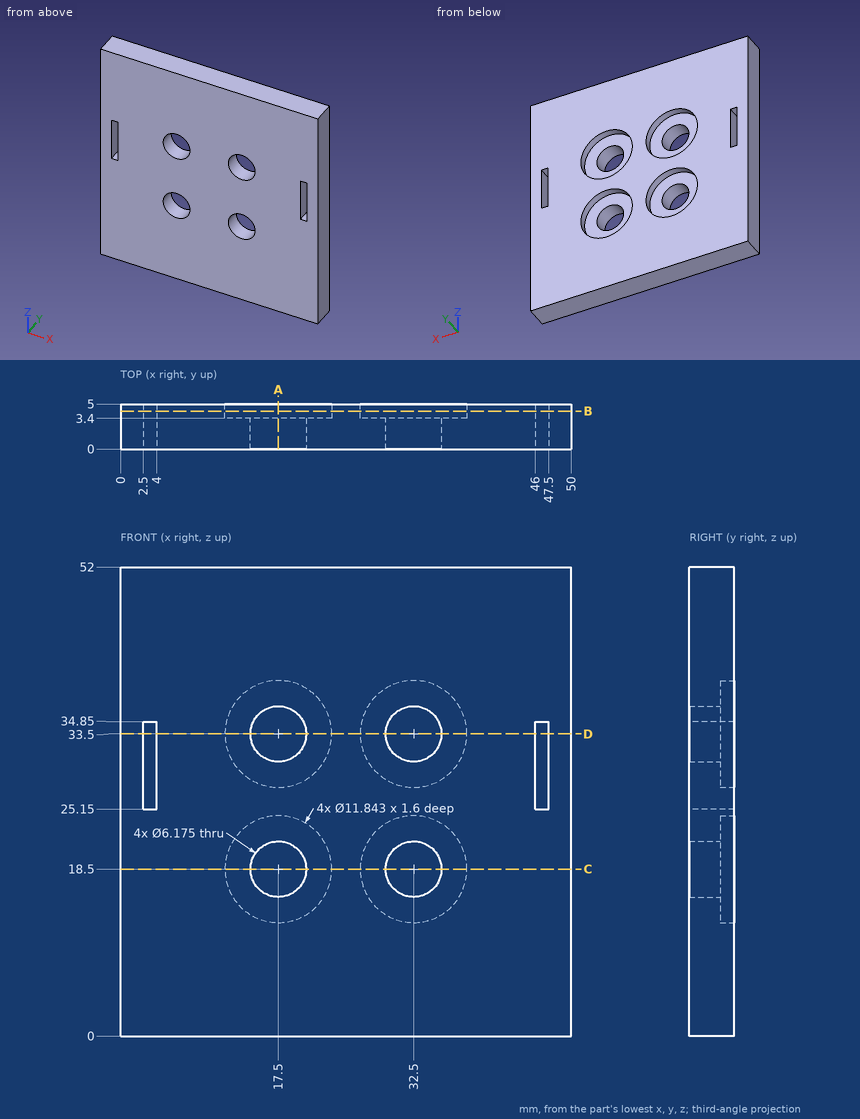
Design review of the part shown in the three views and the two pictorial views. Dimensions are in mm from the part's minimum x, y and z. Round coordinates to 2 decimals unless told otherwise and drop trailing zeros. Order: outer loops, then holes, each group sorted by start corner. A loop starts at its lowest first (then second) coordinate and runs counter-clockwise, first axis right, second up. Notation, with made-up numbers: M 12,-0.5 L 38,-0.5 A11 cw 38,16.5 Z; hole C -36,-32 d8. An arc over 180 degrees is marked long. Put each result on its own line as item: value.
Q1. Consider section A-A (x = 17.5). State the section outline as (y, z) points, and give its area (3 significant figures).
Reported:
outline: M 0,0 L 5,0 L 5,12.58 L 3.4,12.58 L 3.4,15.41 L 0,15.41 Z; M 0,21.59 L 3.4,21.59 L 3.4,24.42 L 5,24.42 L 5,27.58 L 3.4,27.58 L 3.4,30.41 L 0,30.41 Z; M 0,36.59 L 3.4,36.59 L 3.4,39.42 L 5,39.42 L 5,52 L 0,52 Z
area: 180 mm²
Q2. Consider section D-D (z = 33.5). State the section outline as (x, y) points, and give its area (3 significant figures).
Reported:
outline: M 0,0 L 2.5,0 L 2.5,5 L 0,5 Z; M 4,0 L 14.41,0 L 14.41,3.4 L 11.58,3.4 L 11.58,5 L 4,5 Z; M 20.59,0 L 29.41,0 L 29.41,3.4 L 26.58,3.4 L 26.58,5 L 23.42,5 L 23.42,3.4 L 20.59,3.4 Z; M 35.59,0 L 46,0 L 46,5 L 38.42,5 L 38.42,3.4 L 35.59,3.4 Z; M 47.5,0 L 50,0 L 50,5 L 47.5,5 Z
area: 155 mm²
Q3. Insertion check: pin 1 Ø10 at (x, z) = (17.5, 18.5) entering from +Y; pin 2 Ø5 at (x, z) = (32.5, 33.5) entering from -Y. Each pin has a flat end and moves straight along its axis. Give the tip position at first contact, or say it passes through.
Reported:
pin 1: y = 3.4
pin 2: through
Q4. To check wall thickness, follow line 1 (Z direction, x = 17.5, y = 1.45); line 2 (X direction, y = 2.5, z = 18.5); line 3 (X direction, y = 1.9, z = 33.5). State the ranges of each line that lie inside material, in increasing order.
Reported:
line 1: 0 to 15.41, 21.59 to 30.41, 36.59 to 52
line 2: 0 to 14.41, 20.59 to 29.41, 35.59 to 50
line 3: 0 to 2.5, 4 to 14.41, 20.59 to 29.41, 35.59 to 46, 47.5 to 50
Q5. Consider section C-C (z = 18.5). State the section outline as (x, y) points.
Reported:
outline: M 0,0 L 14.41,0 L 14.41,3.4 L 11.58,3.4 L 11.58,5 L 0,5 Z; M 20.59,0 L 29.41,0 L 29.41,3.4 L 26.58,3.4 L 26.58,5 L 23.42,5 L 23.42,3.4 L 20.59,3.4 Z; M 35.59,0 L 50,0 L 50,5 L 38.42,5 L 38.42,3.4 L 35.59,3.4 Z
Q6. Consider section B-B (y = 4.2). State the section outline as (x, z) points, and give its area (3 significant figures).
Reported:
outline: M 0,0 L 50,0 L 50,52 L 0,52 Z; hole M 2.5,25.15 L 4,25.15 L 4,34.85 L 2.5,34.85 Z; hole C 17.5,18.5 d11.84; hole C 17.5,33.5 d11.84; hole C 32.5,18.5 d11.84; hole C 32.5,33.5 d11.84; hole M 46,25.15 L 47.5,25.15 L 47.5,34.85 L 46,34.85 Z
area: 2,130 mm²
